from build123d import *

# Parameters (mm, degrees)
BOSS_EXTRUDE1_DEPTH = 2
SKETCH3_R           = 1.25
CUT_EXTRUDE1_DEPTH  = 2


with BuildPart() as part:
    # Sketch1 → Boss-Extrude1 (new body)
    with BuildSketch(Plane(origin=(0, 0, 0), x_dir=(1, 0, 0), z_dir=(0, 1, 0))):
        Polygon((192.158560219, 82.016387154), (164.708560219, 82.016387154), (164.708560219, 80.016387154), (134.708560219, 80.016387154), (134.708560219, 82.016387154), (104.708560219, 82.016387154), (104.708560219, 80.016387154), (74.708560219, 80.016387154), (74.708560219, 82.016387154), (44.708560219, 82.016387154), (44.708560219, 80.016387154), (14.708560219, 80.016387154), (14.708560219, 82.016387154), (-15.291439781, 82.016387154), (-15.291439781, 80.016387154), (-45.291439781, 80.016387154), (-45.291439781, 82.016387154), (-75.291439781, 82.016387154), (-75.291439781, 80.016387154), (-105.291439781, 80.016387154), (-105.291439781, 82.016387154), (-135.291439781, 82.016387154), (-135.291439781, 80.016387154), (-165.291439781, 80.016387154), (-165.291439781, 82.016387154), (-192.741439781, 82.016387154), (-192.741439781, 80.016387154), (-192.741439781, 52.016387154), (-194.741439781, 52.016387154), (-194.741439781, 22.016387154), (-192.741439781, 22.016387154), (-192.741439781, -7.983612846), (-194.741439781, -7.983612846), (-194.741439781, -37.983612846), (-192.741439781, -37.983612846), (-192.741439781, -65.983612846), (-192.741439781, -67.983612846), (-165.291439781, -67.983612846), (-165.291439781, -65.983612846), (-135.291439781, -65.983612846), (-135.291439781, -67.983612846), (-105.291439781, -67.983612846), (-105.291439781, -65.983612846), (-75.291439781, -65.983612846), (-75.291439781, -67.983612846), (-45.291439781, -67.983612846), (-45.291439781, -65.983612846), (-15.291439781, -65.983612846), (-15.291439781, -67.983612846), (14.708560219, -67.983612846), (14.708560219, -65.983612846), (44.708560219, -65.983612846), (44.708560219, -67.983612846), (74.708560219, -67.983612846), (74.708560219, -65.983612846), (104.708560219, -65.983612846), (104.708560219, -67.983612846), (134.708560219, -67.983612846), (134.708560219, -65.983612846), (164.708560219, -65.983612846), (164.708560219, -67.983612846), (192.158560219, -67.983612846), (192.158560219, -65.983612846), (192.158560219, -37.983612846), (194.158560219, -37.983612846), (194.158560219, -7.983612846), (192.158560219, -7.983612846), (192.158560219, 22.016387154), (194.158560219, 22.016387154), (194.158560219, 52.016387154), (192.158560219, 52.016387154), (192.158560219, 80.016387154), align=None)
    extrude(amount=BOSS_EXTRUDE1_DEPTH)

    # Sketch3 → Cut-Extrude1 (cut)
    with BuildSketch(Plane(origin=(0, 2, 0), x_dir=(1, 0, 0), z_dir=(0, 1, 0))):
        with Locations(Location((-145.841439781, 47.166387154, 0), (0, 0, 270))):
            Circle(SKETCH3_R)
        with Locations(Location((-120.841439781, 47.166387154, 0), (0, 0, 270))):
            Circle(SKETCH3_R)
        with Locations(Location((-105.841439781, 47.166387154, 0), (0, 0, 270))):
            Circle(SKETCH3_R)
        with Locations(Location((-80.841439781, 47.166387154, 0), (0, 0, 270))):
            Circle(SKETCH3_R)
        with Locations(Location((-65.841439781, 47.166387154, 0), (0, 0, 270))):
            Circle(SKETCH3_R)
        with Locations(Location((-40.841439781, 47.166387154, 0), (0, 0, 270))):
            Circle(SKETCH3_R)
        with Locations(Location((-25.841439781, 47.166387154, 0), (0, 0, 270))):
            Circle(SKETCH3_R)
        with Locations(Location((-0.841439781, 47.166387154, 0), (0, 0, 270))):
            Circle(SKETCH3_R)
        with Locations(Location((14.158560219, 47.166387154, 0), (0, 0, 270))):
            Circle(SKETCH3_R)
        with Locations(Location((39.158560219, 47.166387154, 0), (0, 0, 270))):
            Circle(SKETCH3_R)
        with BuildLine():
            Line((-127.466439781, 41.316387154), (-141.741439781, 41.316387154))
            ThreePointArc((-141.741439781, 41.316387154), (-142.448546562, 41.609280373), (-142.741439781, 42.316387154))
            Line((-142.741439781, 42.316387154), (-142.741439781, 52.016387154))
            ThreePointArc((-142.741439781, 52.016387154), (-142.448546562, 52.723493935), (-141.741439781, 53.016387154))
            Line((-141.741439781, 53.016387154), (-127.466439781, 53.016387154))
            ThreePointArc((-127.466439781, 53.016387154), (-124.973888377, 51.983938557), (-123.941439781, 49.491387154))
            Line((-123.941439781, 49.491387154), (-123.941439781, 44.841387154))
            ThreePointArc((-123.941439781, 44.841387154), (-124.973888377, 42.34883575), (-127.466439781, 41.316387154))
        make_face()
        with BuildLine():
            Line((-87.466439781, 41.316387154), (-101.741439781, 41.316387154))
            ThreePointArc((-101.741439781, 41.316387154), (-102.448546562, 41.609280373), (-102.741439781, 42.316387154))
            Line((-102.741439781, 42.316387154), (-102.741439781, 52.016387154))
            ThreePointArc((-102.741439781, 52.016387154), (-102.448546562, 52.723493935), (-101.741439781, 53.016387154))
            Line((-101.741439781, 53.016387154), (-87.466439781, 53.016387154))
            ThreePointArc((-87.466439781, 53.016387154), (-84.973888377, 51.983938557), (-83.941439781, 49.491387154))
            Line((-83.941439781, 49.491387154), (-83.941439781, 44.841387154))
            ThreePointArc((-83.941439781, 44.841387154), (-84.973888377, 42.34883575), (-87.466439781, 41.316387154))
        make_face()
        with BuildLine():
            Line((-47.466439781, 41.316387154), (-61.741439781, 41.316387154))
            ThreePointArc((-61.741439781, 41.316387154), (-62.448546562, 41.609280373), (-62.741439781, 42.316387154))
            Line((-62.741439781, 42.316387154), (-62.741439781, 52.016387154))
            ThreePointArc((-62.741439781, 52.016387154), (-62.448546562, 52.723493935), (-61.741439781, 53.016387154))
            Line((-61.741439781, 53.016387154), (-47.466439781, 53.016387154))
            ThreePointArc((-47.466439781, 53.016387154), (-44.973888377, 51.983938557), (-43.941439781, 49.491387154))
            Line((-43.941439781, 49.491387154), (-43.941439781, 44.841387154))
            ThreePointArc((-43.941439781, 44.841387154), (-44.973888377, 42.34883575), (-47.466439781, 41.316387154))
        make_face()
        with BuildLine():
            Line((-7.466439781, 41.316387154), (-21.741439781, 41.316387154))
            ThreePointArc((-21.741439781, 41.316387154), (-22.448546562, 41.609280373), (-22.741439781, 42.316387154))
            Line((-22.741439781, 42.316387154), (-22.741439781, 52.016387154))
            ThreePointArc((-22.741439781, 52.016387154), (-22.448546562, 52.723493935), (-21.741439781, 53.016387154))
            Line((-21.741439781, 53.016387154), (-7.466439781, 53.016387154))
            ThreePointArc((-7.466439781, 53.016387154), (-4.973888377, 51.983938557), (-3.941439781, 49.491387154))
            Line((-3.941439781, 49.491387154), (-3.941439781, 44.841387154))
            ThreePointArc((-3.941439781, 44.841387154), (-4.973888377, 42.34883575), (-7.466439781, 41.316387154))
        make_face()
        with BuildLine():
            Line((32.533560219, 41.316387154), (18.258560219, 41.316387154))
            ThreePointArc((18.258560219, 41.316387154), (17.551453438, 41.609280373), (17.258560219, 42.316387154))
            Line((17.258560219, 42.316387154), (17.258560219, 52.016387154))
            ThreePointArc((17.258560219, 52.016387154), (17.551453438, 52.723493935), (18.258560219, 53.016387154))
            Line((18.258560219, 53.016387154), (32.533560219, 53.016387154))
            ThreePointArc((32.533560219, 53.016387154), (35.026111623, 51.983938557), (36.058560219, 49.491387154))
            Line((36.058560219, 49.491387154), (36.058560219, 44.841387154))
            ThreePointArc((36.058560219, 44.841387154), (35.026111623, 42.34883575), (32.533560219, 41.316387154))
        make_face()
    extrude(amount=-CUT_EXTRUDE1_DEPTH, mode=Mode.SUBTRACT)


solid = part.part
For this review, take the finished solid that the model builds, in its own axes (mm). Give positions to 0.01 mm unless a question says otherwise; leave off trailing zeros. Loops run counter-clockwise (first coordinate to the right, second up) from the corner with the lowest first, then second, coordinate; pieces in that order, holes last. Notation, with made-up numbers: M -25.75,7 L -6.75,7 A16 ccw -6.75,16 Z; hole C -11.75,85 d9. An arc over 180 degrees is marked long. Answer as a JSON object with one key per item and string values. Group by question number.
Q1. Add section B-B on y = 0.85. Give the number of separate pieces and of enclosed holes in the cut face, and give its area (3 significant figures).
Q2. Insertion check: P1, Ø1, axis at y = 1, z = 67, coming from the +X side; P2, Ø1, axis at y = 0.5, z = 66.5, coming from the -X side; P3, Ø0.6, axis at x = -28, y = 0.5, coming from the +Z side. Each pin has a flat end and moves straight along its axis. Give the tip position at first contact, or say it passes through.
Q3. For probe 1 along X at (y, z) = (1.2, -50); probe 2 along Z at (x, y) = (-135.5, 0.3); probe 3 along X at (y, z) = (0.3, -49), list the stretches that pass through material, from the lowest coordinate up. Write a range as [from, to].
Q4. Add section C-C on x = 157. Give the boundary of the cut face in (y, z).
Q5. Add section A-A on x = 22.5. Give the boundary of the cut face in (y, z), and give its area (3 significant figures).
Checked values:
{
 "1": {"separate pieces": "1", "enclosed holes": "15", "area": "56,100 mm²"},
 "2": {"P1": "x = 192.16", "P2": "x = -192.74", "P3": "z = 65.98"},
 "3": {"probe 1": "[-194.74, -142.74], [-123.98, -102.74], [-83.98, -62.74], [-43.98, -22.74], [-3.98, 17.26], [36.02, 194.16]", "probe 2": "[-80.02, -53.02], [-41.32, 65.98]", "probe 3": "[-194.74, -142.74], [-123.94, -102.74], [-83.94, -62.74], [-43.94, -22.74], [-3.94, 17.26], [36.06, 194.16]"},
 "4": {"outline": "M 0,-80.02 L 2,-80.02 L 2,65.98 L 0,65.98 Z"},
 "5": {"outline": "M 0,-80.02 L 2,-80.02 L 2,-53.02 L 0,-53.02 Z; M 0,-41.32 L 2,-41.32 L 2,65.98 L 0,65.98 Z", "area": "269 mm²"}
}
